from build123d import *

# Parameters (mm, degrees)
SKICA1_R                 = 1.65
P_IDAT_VYSUNUT_M1_DEPTH  = 20
SKICA2_R                 = 3
P_IDAT_VYSUNUT_M2_DEPTH  = 2.5
SKICA4_R                 = 1.65
ODEBRAT_VYSUNUT_M1_DEPTH = 5


with BuildPart() as part:
    # Skica1 → Přidat vysunutím1 (new body)
    with BuildSketch(Plane.XY):
        Circle(SKICA1_R)
    extrude(amount=P_IDAT_VYSUNUT_M1_DEPTH)

    # Skica2 → Přidat vysunutím2 (add, symmetric)
    with BuildSketch(Plane(origin=(0, 0, 0), x_dir=(1, 0, 0), z_dir=(0, 1, 0))):
        with Locations((0, 2)):
            Circle(SKICA2_R)
    extrude(amount=P_IDAT_VYSUNUT_M2_DEPTH, both=True)

    # Skica4 → Odebrat vysunutím1 (cut)
    with BuildSketch(Plane(origin=(0, 2.5, 0), x_dir=(1, 0, 0), z_dir=(0, 1, 0))):
        with Locations((0, 2.001079416)):
            Circle(SKICA4_R)
    extrude(amount=-ODEBRAT_VYSUNUT_M1_DEPTH, mode=Mode.SUBTRACT)


solid = part.part
Source: CAD feature listing. Evaluate the final solid. Frame: model axes, mm. A direction names the side the tool comes from. Round coordinates to 2 decimals unless told otherwise and drop trailing zeros. Write each loop counter-clockwise with the first axis right and the second up, starting at its lowest first coordinate (ties: lowest second). Pieces come first, ordered by that corner, then holes. Notation, with made-up numbers: (89.5, -24.5) - (98.5, -24.5) arc R33 cw to (98.5, 5.5) - close; hole circle Ø3 at (32, 34.5). An arc over 180 degrees is marked (long way). Use CSV: the item, a comma, the result in double quotes. Start each with the question number.
(1) Set-up query: faces 4 (the face through (-1.216, 1.115, 10.116)), 5 (the face through (1.3, 2.5, -0.7)). Return all of +Z, -Z, +X, -X, +Y, -Y with unobstructed straight access to the full face (end or side cutting, diameter ignored); none if empty.
(2) Cut plane A-A, the plane x = 0. Return loops of the section in (y, z), and give its area (3 significant figures).
(3) Mould query, pull axis X, two halves, no side actions, for faces 1 (the face through (0, 0, 20)), 2 (the face through (-0.4, 0, -0.4)), 3 (the face through (0, 0, -5)). Classes: pulls with the +X half, pulls with the -X half, needs draft (parallel to the pull), parting line crosses it, or undercut.
(4) Cut plane C-C, the plane z = 10. Return loops of the section in (x, y), and give its area (3 significant figures).
(5) First-contact query: pin 1 Ø2 at (x, y) = (-1.5, 1.5) entering from -Z; pin 2 Ø1 at (x, z) = (1, 15.5) entering from +Y. Flat tips, straight axial feed; report the tip coordinate or a pass-through.
(6) Material intervals for probe 1 along Z at (x, y) = (0, 0.6); probe 2 along Z at (x, y) = (-1, -0.65); probe 3 along X at (y, z) = (-0.05, 8.5), sorted ascending. Write a range as [from, to].
(7) Cut plane B-B, the plane y = 0.55. Return loops of the section in (x, z).
Geometry says:
1,face 4,"+Z"
1,face 5,"+Z, -Z, +X, -X, +Y"
2,outline,"(-2.5, -5) - (2.5, -5) - (2.5, -3.65) - (-2.5, -3.65) - close; (-2.5, -0.35) - (2.5, -0.35) - (2.5, 1) - (1.65, 1) - (1.65, 20) - (-1.65, 20) - (-1.65, 1) - (-2.5, 1) - close"
2,area,"76.2 mm²"
3,face 1,"needs draft"
3,face 2,"undercut"
3,face 3,"parting line crosses it"
4,outline,"circle Ø3.3 at (0, 0)"
4,area,"8.55 mm²"
5,pin 1,"z = -4.96"
5,pin 2,"y = 1.57"
6,probe 1,"[-5, -3.65], [-0.35, 20]"
6,probe 2,"[-4.83, -3.31], [-0.69, 20]"
6,probe 3,"[-1.65, 1.65]"
7,outline,"(-1.56, 0.57) arc R3 ccw (long way) to (1.56, 0.57) - (1.56, 20) - (-1.56, 20) - close; hole circle Ø3.3 at (0, -2)"
